The listing builds one solid part. Answer for the finished solid, in the listing's coordinates (mm). Coordinates: 2 decimals unless noted, no trailing zeros. Order: outer loops, then holes, each group sorted by start corner. A loop starts at its lowest first (then second) coordinate and runs counter-clockwise, first axis right, second up.
Autodesk Inventor part; units mm, degrees
ref_plane "YZ Plane" through (0, 0, 0) normal (1, 0, 0) x (0, 1, 0)
ref_plane "XZ Plane" through (0, 0, 0) normal (0, 1, 0) x (-1, 0, 0)
ref_plane "XY Plane" through (0, 0, 0) normal (0, 0, 1) x (1, 0, 0)
sketch "Sketch1" plane through (0, 0, 0) normal (0, 1, 0) x (-1, 0, 0)
  circle A0 centre (0, 0) radius 47.625
  circle A1 centre (0, 0) radius 41.275 construction
  point P0 (41.275, 0)
  point P1 (0, -41.275)
  point P2 (-41.275, 0)
  point P3 (0, 41.275)
  dimension "d0" = 95.25
  dimension "d1" = 82.55
extrude "Extrusion1" add sketch "Sketch1" against normal blind 31.75
hole "Hole1" at (-41.275, 0, 0) at (0, 0, -41.275) at (41.275, 0, 0) at (0, 0, 41.275) direction (0, -1, 0) diameter 4.4958 end through all
sketch "Sketch2" plane through (0, 0, 0) normal (0, 1, 0) x (1, 0, 0)
  point P0 (0, 0)
  point P1 (-0.2961, 4.5812)
hole "Hole2" at (0, 0, 0) direction (0, -1, 0) diameter 69.85 end through all
sketch "Sketch3" plane through (0, -31.75, 0) normal (0, -1, 0) x (1, 0, 0)
  circle A0 centre (0, 41.275) radius 2.2479
  circle A1 centre (-41.275, 0) radius 2.2479
  circle A2 centre (0, -41.275) radius 2.2479
  circle A3 centre (41.275, 0) radius 2.2479
  circle A4 centre (0, 41.275) radius 7.62
  circle A5 centre (-41.275, 0) radius 7.62
  circle A6 centre (0, -41.275) radius 7.62
  circle A7 centre (41.275, 0) radius 7.62
  point P0 (0, 0)
  dimension "d18" = 15.24
properties material "ABS, BLACK"
(1) Consider line 1 (Z direction, x = 0, y = -14) (3 decimals); line 2 (Z direction, x = -15.5, y = -7); line 3 (X direction, y = -6, z = 1). Determine where each line is inside the solid, lowest interval first.
(2) Find section B-B (z = 41.5). Write down the section's boundary in (x, y).
(3) Find section C-C (z = 0). Write down the section's boundary in (x, y) (3 decimals), and give its area (3 significant figures).
(4) Find section D-D (x = -11.5). Write down the section's boundary in (y, z).
(5) Find section A-A (x = 0). Write down the section's boundary in (y, z) (3 decimals).
(6) The mould has two halves that part along X. Classify faces 1 (the face through (0.86, -16.1, 43.35)), 2 (the face through (37.794, -15.653, -28.979)), 3 (the face through (-3, -31.75, 36)), 4 (the face through (39.046, -16.097, -0.293)): released by +X, released by -X, zero draft, split by the parting line, or undercut.
(7) Each of these flat-tipped pins is pushed along its axis until it touches: pin 1 Ø2.5 at (x, z) = (0, -41.275) entering from +Y; pin 2 Ø1 at (y, z) = (-3.5, 29.5) entering from +X; pin 3 Ø3 at (y, z) = (-26, -28.5) entering from -X; pin 4 Ø5 at (x, z) = (0, 41.275) entering from +Y. Where does it stop, or does it pass through?
Findings below:
1. line 1: z = -47.625 to -43.523, -39.027 to -34.925, 34.925 to 39.027, 43.523 to 47.625
1. line 2: z = -45.03 to -31.3, 31.3 to 45.03
1. line 3: x = -47.61 to -43.29, -39.26 to -34.91, 34.91 to 39.26, 43.29 to 47.61
2. outline: (-23.36, -31.75) - (-2.24, -31.75) - (-2.24, 0) - (-23.36, 0) - close; (2.24, -31.75) - (23.36, -31.75) - (23.36, 0) - (2.24, 0) - close
3. outline: (-47.625, -31.75) - (-43.523, -31.75) - (-43.523, 0) - (-47.625, 0) - close; (-39.027, -31.75) - (-34.925, -31.75) - (-34.925, 0) - (-39.027, 0) - close; (34.925, -31.75) - (39.027, -31.75) - (39.027, 0) - (34.925, 0) - close; (43.523, -31.75) - (47.625, -31.75) - (47.625, 0) - (43.523, 0) - close
3. area: 521 mm2
4. outline: (-31.75, -46.22) - (0, -46.22) - (0, -32.98) - (-31.75, -32.98) - close; (-31.75, 32.98) - (0, 32.98) - (0, 46.22) - (-31.75, 46.22) - close
5. outline: (-31.75, -47.625) - (0, -47.625) - (0, -43.523) - (-31.75, -43.523) - close; (-31.75, -39.027) - (0, -39.027) - (0, -34.925) - (-31.75, -34.925) - close; (-31.75, 34.925) - (0, 34.925) - (0, 39.027) - (-31.75, 39.027) - close; (-31.75, 43.523) - (0, 43.523) - (0, 47.625) - (-31.75, 47.625) - close
6. face 1: undercut
6. face 2: split by the parting line
6. face 3: zero draft
6. face 4: undercut
7. pin 1: passes through
7. pin 2: stops at x = 37.78
7. pin 3: stops at x = -39.23
7. pin 4: stops at y = 0
